Autodesk Fusion 360 part; units mm, degrees
sketch "Sketch1" plane through (0, 0, 0) normal (1, 0, 0) x (0, 1, 0)
  line L0 (25.4, 0) -> (25.4, -3.175)
  line L1 (12.7, 0) -> (12.7, -3.175)
  line L2 (76.2, 25.4) -> (76.2, 12.7)
  line L3 (0, 0) -> (0, 25.4)
  line L4 (0, 12.7) -> (-3.175, 12.7)
  line L5 (76.2, 12.7) -> (79.375, 12.7)
  line L6 (-3.175, 25.4) -> (0, 25.4)
  line L7 (63.5, -3.175) -> (63.5, 0)
  line L8 (50.8, 0) -> (50.8, -3.175)
  line L9 (79.375, 12.7) -> (79.375, 25.4)
  line L10 (0, -3.175) -> (0, 0)
  line L11 (0, 0) -> (0, 12.7)
  line L12 (25.4, -3.175) -> (38.1, -3.175)
  line L13 (-3.175, 12.7) -> (-3.175, 25.4)
  line L14 (79.375, 25.4) -> (76.2, 25.4)
  line L15 (0, 0) -> (-7.62, 0)
  line L16 (0, 0) -> (-5.715, 0)
  line L17 (-5.715, 0) -> (-5.715, 38.1)
  line L18 (-5.715, 38.1) -> (-5.715, 43.815)
  line L19 (-5.715, 43.815) -> (76.2, 43.815)
  line L20 (76.2, 43.815) -> (81.915, 43.815)
  line L21 (81.915, 43.815) -> (81.915, 0)
  line L22 (81.915, 0) -> (81.915, -5.715)
  line L23 (81.915, -5.715) -> (0, -5.715)
  line L24 (0, -5.715) -> (-5.715, -5.715)
  line L25 (-5.715, -5.715) -> (-5.715, 0)
  line L26 (-5.715, 43.815) -> (12.7, 43.815)
  line L27 (12.7, 43.815) -> (12.7, 40.64)
  line L28 (12.7, 40.64) -> (12.7, 27.94)
  line L29 (81.915, 43.815) -> (63.5, 43.815)
  line L30 (63.5, 43.815) -> (63.5, 27.94)
  line L31 (63.5, 27.94) -> (12.7, 27.94)
  line L32 (12.7, 40.64) -> (63.5, 40.64)
  line L33 (63.5, -3.175) -> (50.8, -3.175)
  line L34 (63.5, 0) -> (50.8, 0)
  line L35 (25.4, -3.175) -> (12.7, -3.175)
  line L36 (12.7, 0) -> (25.4, 0)
  dimension "d2" = 12.7
  dimension "d3" = 3.175
  dimension "d4" = 12.7
  dimension "d6" = 12.7
  dimension "d9" = 12.7
  dimension "d10" = 3.175
  dimension "d12" = 12.7
  dimension "d13" = 3.175
  dimension "d14" = 12.7
  dimension "d16" = 3.175
  dimension "d17" = 12.7
  dimension "d18" = 7.62
  dimension "d21" = 5.715
  dimension "d22" = 5.715
  dimension "d23" = 5.715
  dimension "d24" = 5.715
  dimension "d25" = 3.175
  dimension "d26" = 12.7
  dimension "d27" = 18.415
extrude "Extrude1" add sketch "Sketch1" along normal blind 3.175 contours L17 L18 L19 L20 L21 L22 L23 L24 L25 L26 L27 L28 L29 L30 L31 | L19 L27 L30 L32
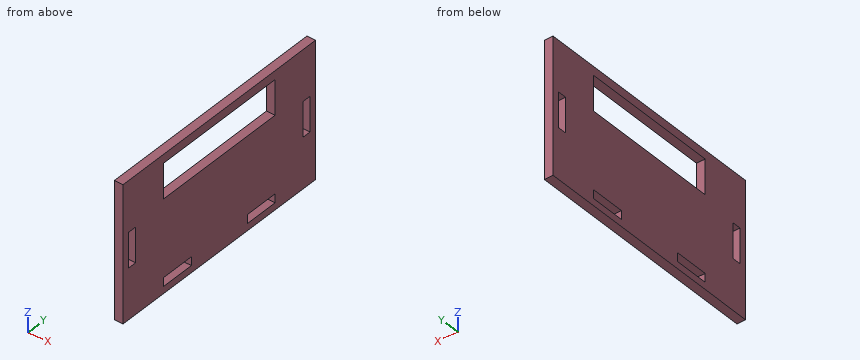
Check sheet for the modelled part. Datum: model origin and axes. Units: mm. Round coordinates to 2 decimals unless told otherwise and drop trailing zeros. Loops run counter-clockwise (first coordinate to the right, second up) from the corner with the lowest first, then second, coordinate; pieces in that order, holes last. Notation, with made-up numbers: (81, -26.75) -> (131, -26.75) arc R36 ccw to (131, 8.25) -> close; hole circle Ø1 at (65, 67.25). An arc over 180 degrees is marked (long way). Put each result on its own line as item: value. Start each with the question number.
1. Section check D-D (x = 2.65). Enter the section's corners in (y, z) (3 decimals).
2. Section check B-B (z = -1.5). Enter the section's corners in (x, y) (3 decimals), plus the area to 3 significant figures.
3. Section check A-A (z = 34). Enter the section's corners in (x, y) (3 decimals), plus the area to 3 significant figures.
4. Section check C-C (y = 41.5). Enter the section's corners in (x, z) (3 decimals), plus the area to 3 significant figures.
5. Scan lines: probe 1 along Z at (x, y) = (2.1, 51) (3 decimals); probe 2 along Y at (x, z) = (2.1, 23.5) (3 decimals); probe 3 along Y at (x, z) = (2.35, -2.5) (3 decimals). Record each from-to range of solid material in increasing order.
Findings:
1. outline: (-5.715, -5.715) -> (81.915, -5.715) -> (81.915, 43.815) -> (-5.715, 43.815) -> close; hole (-3.175, 12.7) -> (0, 12.7) -> (0, 25.4) -> (-3.175, 25.4) -> close; hole (12.7, -3.175) -> (25.4, -3.175) -> (25.4, 0) -> (12.7, 0) -> close; hole (12.7, 27.94) -> (63.5, 27.94) -> (63.5, 40.64) -> (12.7, 40.64) -> close; hole (50.8, -3.175) -> (63.5, -3.175) -> (63.5, 0) -> (50.8, 0) -> close; hole (76.2, 12.7) -> (79.375, 12.7) -> (79.375, 25.4) -> (76.2, 25.4) -> close
2. outline: (0, -5.715) -> (3.175, -5.715) -> (3.175, 12.7) -> (0, 12.7) -> close; (0, 25.4) -> (3.175, 25.4) -> (3.175, 50.8) -> (0, 50.8) -> close; (0, 63.5) -> (3.175, 63.5) -> (3.175, 81.915) -> (0, 81.915) -> close
2. area: 198 mm^2
3. outline: (0, -5.715) -> (3.175, -5.715) -> (3.175, 12.7) -> (0, 12.7) -> close; (0, 63.5) -> (3.175, 63.5) -> (3.175, 81.915) -> (0, 81.915) -> close
3. area: 117 mm^2
4. outline: (0, -5.715) -> (3.175, -5.715) -> (3.175, 27.94) -> (0, 27.94) -> close; (0, 40.64) -> (3.175, 40.64) -> (3.175, 43.815) -> (0, 43.815) -> close
4. area: 117 mm^2
5. probe 1: z = -5.715 to -3.175, 0 to 27.94, 40.64 to 43.815
5. probe 2: y = -5.715 to -3.175, 0 to 76.2, 79.375 to 81.915
5. probe 3: y = -5.715 to 12.7, 25.4 to 50.8, 63.5 to 81.915
